Can you work these out from the model? Positions are in its coordinate system, mm. A direction names the side the tool comes from. Give positions to 0.01 mm unless a question says otherwise; leave off trailing zeros. Order: outer loops, then holes, each group sorted by start corner. A loop starts at its lowest first (then second) coordinate and runs counter-clockwise, first axis right, second up. Notation, with made-up numbers: M 16,29 L 50,29 A25 cw 50,68 Z; hole C 82.25,24 d4. An arc over 180 degrees is marked long. One line per question, with ' | ' between items. Start each with the question number.
1) If we section it at C-C, the plane y = 0: Please give me the cut outline in (x, z), plus the area to 3 significant figures.
2) Please list where these lines run through material, in increasing order: line 1 along X through (y, z) = (0.25, -1); line 2 along Z through (x, y) = (10, -1.25); line 3 along Z through (x, y) = (14.5, -1.5). Write a range as [from, to].
3) I'm going to push flat-ended pins straight in: pin 1 Ø1 at (x, z) = (-6, 9.5) entering from -Y; pin 2 Ø3 at (y, z) = (0.5, 7.5) entering from +X; pin 3 Ø1.5 at (x, z) = (4.5, 7) entering from +Y; pin 4 Ø1.9 at (x, y) = (15.43, 0) entering from +Z. Where does each tip first touch, or does it pass through?
4) If we section it at A-A, the plane z = -1.25: Please give me the cut outline in (x, y).
5) If we section it at B-B, the plane x = -16: Please give me the cut outline in (y, z), plus the area to 3 significant figures.
6) If we section it at D-D, the plane z = 8.25: Please give me the cut outline in (x, y), plus the area to 3 significant figures.
7) For faces 1 (the cylindrical face through (-10.269, 2.366, 11.634)), 2 (the flat face through (0, 2.578, 12)), 3 (the flat face through (11.55, 0.52, 11.63)), which set-ups out of +Z, -Z, +X, -X, +Y, -Y let a thin tool reach every point of the face, with its end or its side?
```python
from build123d import *

# Parameters (mm, degrees)
F0_R     = 1.1684
F1_DEPTH = 4.5085
F3_DEPTH = 4.953
F5_DEPTH = 4.4069
F6_R     = 0.254
F7_DEPTH = 3.81


with BuildPart() as f1:
    # F0 (on Top) → F1 (new body, symmetric)
    with BuildSketch(Plane.XY):
        with BuildLine():
            Line((16.6497, 4.4577), (-16.6497, 4.4577))
            ThreePointArc((-16.6497, 4.4577), (-17.763252, 3.996452), (-18.2245, 2.8829))
            Line((-18.2245, 2.8829), (-18.2245, -2.8829))
            ThreePointArc((-18.2245, -2.8829), (-17.763252, -3.996452), (-16.6497, -4.4577))
            Line((-16.6497, -4.4577), (16.6497, -4.4577))
            ThreePointArc((16.6497, -4.4577), (17.763252, -3.996452), (18.2245, -2.8829))
            Line((18.2245, -2.8829), (18.2245, 2.8829))
            ThreePointArc((18.2245, 2.8829), (17.763252, 3.996452), (16.6497, 4.4577))
        make_face()
        with Locations((-15.4305, 0)):
            Circle(F0_R, mode=Mode.SUBTRACT)
        with Locations((15.4305, 0)):
            Circle(F0_R, mode=Mode.SUBTRACT)
    extrude(amount=F1_DEPTH, both=True)

    # F2 (on face) → F3 (join)
    with BuildSketch(Plane.XY.offset(4.5085)):
        with BuildLine():
            Line((-11.13142, -2.8956), (11.132878, -2.8956))
            ThreePointArc((11.132878, -2.8956), (12.489771, -2.120071), (12.510229, -0.557322))
            Line((12.510229, -0.557322), (11.045966, 2.084278))
            ThreePointArc((11.045966, 2.084278), (10.467886, 2.677694), (9.668615, 2.8956))
            Line((9.668615, 2.8956), (-9.667157, 2.8956))
            ThreePointArc((-9.667157, 2.8956), (-10.466429, 2.677694), (-11.044508, 2.084278))
            Line((-11.044508, 2.084278), (-12.508771, -0.557322))
            ThreePointArc((-12.508771, -0.557322), (-12.488314, -2.120071), (-11.13142, -2.8956))
        make_face()
    extrude(amount=F3_DEPTH)

    # F4 (on face) → F5 (join)
    with BuildSketch(Plane.XY.offset(9.4615)):
        with BuildLine():
            Line((9.481593, 2.5781), (-9.480136, 2.5781))
            ThreePointArc((-9.480136, 2.5781), (-10.279407, 2.360194), (-10.857487, 1.766778))
            Line((-10.857487, 1.766778), (-12.220627, -0.692392))
            ThreePointArc((-12.220627, -0.692392), (-12.204129, -1.952674), (-11.10986, -2.5781))
            Line((-11.10986, -2.5781), (11.111317, -2.5781))
            ThreePointArc((11.111317, -2.5781), (12.205586, -1.952674), (12.222084, -0.692392))
            Line((12.222084, -0.692392), (10.858944, 1.766778))
            ThreePointArc((10.858944, 1.766778), (10.280864, 2.360194), (9.481593, 2.5781))
        make_face()
    extrude(amount=F5_DEPTH)

    # F6 (on face) → F7 (join)
    with BuildSketch(Plane(origin=(0, 0, -4.5085), x_dir=(1, 0, 0), z_dir=(0, 0, -1))):
        with Locations((-12.3825, 2.8575)):
            Circle(F6_R)
        with Locations((-10.4775, 2.8575)):
            Circle(F6_R)
        with Locations((-8.5725, 2.8575)):
            Circle(F6_R)
        with Locations((-6.6675, 2.8575)):
            Circle(F6_R)
        with Locations((-4.7625, 2.8575)):
            Circle(F6_R)
        with Locations((-2.8575, 2.8575)):
            Circle(F6_R)
        with Locations((-0.9525, 2.8575)):
            Circle(F6_R)
        with Locations((0.9525, 2.8575)):
            Circle(F6_R)
        with Locations((2.8575, 2.8575)):
            Circle(F6_R)
        with Locations((4.7625, 2.8575)):
            Circle(F6_R)
        with Locations((6.6675, 2.8575)):
            Circle(F6_R)
        with Locations((8.5725, 2.8575)):
            Circle(F6_R)
        with Locations((10.4775, 2.8575)):
            Circle(F6_R)
        with Locations((12.3825, 2.8575)):
            Circle(F6_R)
        with Locations((-11.43, 0.9525)):
            Circle(F6_R)
        with Locations((-9.525, 0.9525)):
            Circle(F6_R)
        with Locations((-7.62, 0.9525)):
            Circle(F6_R)
        with Locations((-5.715, 0.9525)):
            Circle(F6_R)
        with Locations((-3.81, 0.9525)):
            Circle(F6_R)
        with Locations((-1.905, 0.9525)):
            Circle(F6_R)
        with Locations((-10.4775, -0.9525)):
            Circle(F6_R)
        with Locations((-8.5725, -0.9525)):
            Circle(F6_R)
        with Locations((-6.6675, -0.9525)):
            Circle(F6_R)
        with Locations((-4.7625, -0.9525)):
            Circle(F6_R)
        with Locations((-2.8575, -0.9525)):
            Circle(F6_R)
        with Locations((-0.9525, -0.9525)):
            Circle(F6_R)
        with Locations((9.525, 0.9525)):
            Circle(F6_R)
        with Locations((7.62, 0.9525)):
            Circle(F6_R)
        with Locations((6.6675, -0.9525)):
            Circle(F6_R)
        with Locations((11.43, 0.9525)):
            Circle(F6_R)
        with Locations((4.7625, -0.9525)):
            Circle(F6_R)
        with Locations((2.8575, -0.9525)):
            Circle(F6_R)
        with Locations((5.715, 0.9525)):
            Circle(F6_R)
        with Locations((8.5725, -0.9525)):
            Circle(F6_R)
        with Locations((1.905, 0.9525)):
            Circle(F6_R)
        with Locations((3.81, 0.9525)):
            Circle(F6_R)
        with Locations((10.4775, -0.9525)):
            Circle(F6_R)
        with Locations((0.9525, -0.9525)):
            Circle(F6_R)
        with Locations((-11.43, -2.8575)):
            Circle(F6_R)
        with Locations((-9.525, -2.8575)):
            Circle(F6_R)
        with Locations((-7.62, -2.8575)):
            Circle(F6_R)
        with Locations((-5.715, -2.8575)):
            Circle(F6_R)
        with Locations((-3.81, -2.8575)):
            Circle(F6_R)
        with Locations((-1.905, -2.8575)):
            Circle(F6_R)
        with Locations((0, -2.8575)):
            Circle(F6_R)
        with Locations((1.905, -2.8575)):
            Circle(F6_R)
        with Locations((3.81, -2.8575)):
            Circle(F6_R)
        with Locations((5.715, -2.8575)):
            Circle(F6_R)
        with Locations((7.62, -2.8575)):
            Circle(F6_R)
        with Locations((9.525, -2.8575)):
            Circle(F6_R)
        with Locations((11.43, -2.8575)):
            Circle(F6_R)
    extrude(amount=F7_DEPTH)


solid = f1.part
```
Results found:
1) outline: M -18.22,-4.51 L -16.6,-4.51 L -16.6,4.51 L -18.22,4.51 Z; M -14.26,-4.51 L 14.26,-4.51 L 14.26,4.51 L 12.2,4.51 L 12.2,9.46 L 11.84,9.46 L 11.84,13.87 L -11.84,13.87 L -11.84,9.46 L -12.2,9.46 L -12.2,4.51 L -14.26,4.51 Z; M 16.6,-4.51 L 18.22,-4.51 L 18.22,4.51 L 16.6,4.51 Z | area: 512 mm²
2) line 1: x = [-18.22, -16.57], [-14.29, 14.29], [16.57, 18.22] | line 2: z = [-4.51, 13.87] | line 3: z = [-4.51, 4.51]
3) pin 1: stops at y = -2.9 | pin 2: stops at x = 12.67 | pin 3: stops at y = 2.9 | pin 4: passes through
4) outline: M -18.22,-2.88 A1.57 ccw -16.65,-4.46 L 16.65,-4.46 A1.57 ccw 18.22,-2.88 L 18.22,2.88 A1.57 ccw 16.65,4.46 L -16.65,4.46 A1.57 ccw -18.22,2.88 Z; hole C -15.43,0 d2.34; hole C 15.43,0 d2.34
5) outline: M -4.46,-4.51 L -1.02,-4.51 L -1.02,4.51 L -4.46,4.51 Z; M 1.02,-4.51 L 4.46,-4.51 L 4.46,4.51 L 1.02,4.51 Z | area: 62.0 mm²
6) outline: M -12.51,-0.56 A1.57 ccw -11.13,-2.9 L 11.13,-2.9 A1.57 ccw 12.51,-0.56 L 11.05,2.08 A1.57 ccw 9.67,2.9 L -9.67,2.9 A1.57 ccw -11.04,2.08 Z | area: 138 mm²
7) face 1: +Z, -X, +Y | face 2: +Z, +X, -X, +Y | face 3: +Z, +X, +Y
